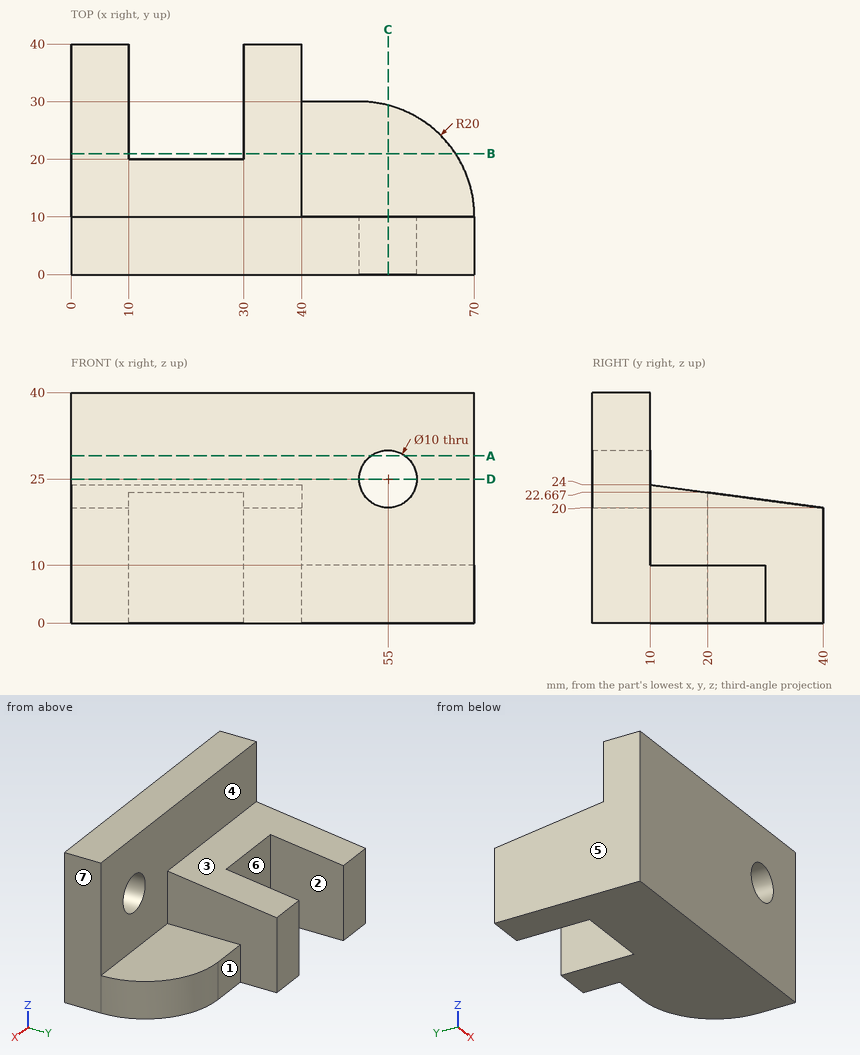
Answer from the drawing. Dimensions are ordinates in mm from the lowest x, y and z of the part. A direction names the side the tool comes from. Give positions to 0.01 mm unless a question says otherwise; leave off trailing zeros. Write each loop counter-clockwise with the first axis right and the second up, starting at its lowest first coordinate (ties: lowest second). Pieces come first, ordered by that corner, then holes. Notation, with made-up numbers: M 83.25,-18 L 100.25,-18 A19 cw 100.25,-1 Z; hole C -14.75,26 d11. An arc over 180 degrees is marked long. Answer as CSV lines item,"result".
Q1. A cutting plane is placed at B-B on y = 21. Write down the section's boundary in (x, z), plus the area to 3 significant figures.
A:
outline,"M 0,0 L 10,0 L 10,22.53 L 0,22.53 Z; M 30,0 L 66.7,0 L 66.7,10 L 40,10 L 40,22.53 L 30,22.53 Z"
area,"718 mm²"
Q2. The mould has two halves that part along X. Classify the marked faces 5, 6 and 7: +X half, -X half, draft (parallel to the pull), parting line (faces both ways), or undercut.
A:
face 5,"-X half"
face 6,"undercut"
face 7,"+X half"
Q3. A cutting plane is placed at D-D on z = 25. Write down the section's boundary in (x, y).
A:
outline,"M 0,0 L 50,0 L 50,10 L 0,10 Z; M 60,0 L 70,0 L 70,10 L 60,10 Z"
Q4. A tool of negligible diameter and unlimited length cuts with its end or side. For the marked faces 1, 2, 3 and 4, from which of +Z, -Z, +X, -X, +Y, -Y can it reach the whole face along a straight path? Write none if from no direction.
A:
face 1,"+Z, -Z, +X, +Y"
face 2,"+Z, -Z, +Y"
face 3,"+Z, +X, -X, +Y"
face 4,"+Z, +X, +Y"
Q5. A cutting plane is placed at C-C on x = 55. Write down the section's boundary in (y, z) (1 decimal), plus the area to 3 significant figures.
A:
outline,"M 0,0 L 29.4,0 L 29.4,10 L 10,10 L 10,20 L 0,20 Z; M 0,30 L 10,30 L 10,40 L 0,40 Z"
area,"494 mm²"
Q6. A cutting plane is placed at A-A on z = 29. Write down the section's boundary in (x, y), plus the area to 3 significant figures.
A:
outline,"M 0,0 L 52,0 L 52,10 L 0,10 Z; M 58,0 L 70,0 L 70,10 L 58,10 Z"
area,"640 mm²"
Q7. Given P1, Ø1, axis at y = 31, z = 20, coming from the +X side; P2, Ø16, axis at x = 50, y = 20, coming from the +Z side; P3, Ø19, axis at y = 28, z = 6.5, coming from the +X side, each flat-ended and moving along its own axis, determine where each tip first touches the part or whether it passes through.
A:
P1,"stops at x = 40"
P2,"stops at z = 10"
P3,"stops at x = 68.1"
Q8. Find the intervals of material crossed by probe 1 along X at (y, z) = (6.25, 25); probe 2 along Z at (x, y) = (55, 4); probe 3 along X at (y, z) = (28, 19.5), in increasing order. Write a range as [from, to].
A:
probe 1,"x = [0, 50], [60, 70]"
probe 2,"z = [0, 20], [30, 40]"
probe 3,"x = [0, 10], [30, 40]"
